Model file for the job. Use its own axes, mm. Face numbers are marked on the shaded views. A direction names the side the tool comes from. Round coordinates to 2 decimals unless told otherwise and drop trailing zeros. Order: outer loops, then holes, each group sorted by start corner. A loop starts at its lowest first (then second) coordinate and runs counter-clockwise, first axis right, second up. Notation, with made-up numbers: M -16,-15.75 L 11,-15.75 A22 cw 11,6.25 Z; hole C 85,12.25 d7. An arc over 180 degrees is marked long. Return JSON: item names as keys, results as strings. Group by question number.
Item 1: Slice it at C-C on x = 15.25. Write the cut outline in (y, z) (3 decimals), then the cut area to 3 significant figures.
Item 2: Pull direction Z, two halves, no side cores. Call the marked faces 1, 2 and 3: pulls with the +Z half, pulls with the -Z half, needs draft (parallel to the pull), parting line crosses it, or undercut.
Item 3: Pin check, flat tips, straight feed: pin 1 Ø1 at (x, y) = (7, -11.5) entering from +Z; pin 2 Ø0.7 at (x, y) = (8.5, 12) entering from +Z; pin 3 Ø2 at (x, z) = (14.5, 8.5) entering from -Y. Stop position of each tip, or through.
Item 4: Slice it at B-B on z = 0. Write the cut outline in (x, y).
Item 5: Slice it at A-A on y = 0. Write the cut outline in (x, z), then the cut area to 3 significant figures.
Item 6: Which spindle directions (+Z, -Z, +X, -X, +Y, -Y) get a long thin tool onto all of the face, cutting with end or side? Do the marked faces 4 and 5. Say none if no direction does.
Item 7: Probe line 1 along Z through (x, y) = (15.25, -8); line 2 along Z through (x, y) = (6.5, 11.5) (3 decimals); line 3 along Z through (x, y) = (12.25, -10). List the from-to ranges inside material, lowest first.
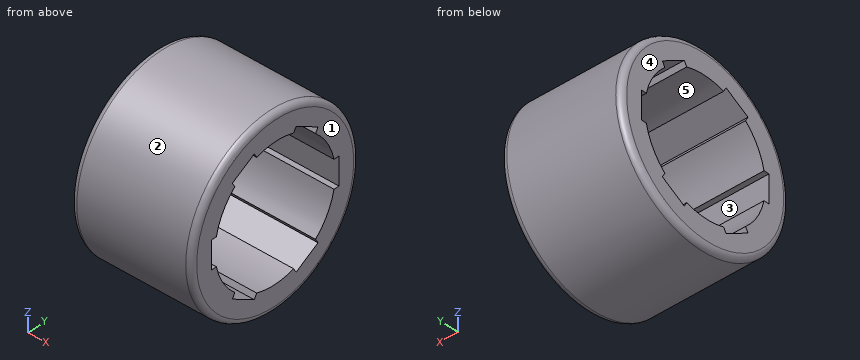
from build123d import *

# Parameters (mm, degrees)
CROQUIS1_R              = 16
SALIENTE_EXTRUIR1_DEPTH = 21
REDONDEO1_R             = 1


with BuildPart() as part:
    # Croquis1 → Saliente-Extruir1 (new body)
    with BuildSketch(Plane(origin=(0, 0, 0), x_dir=(0, 0, -1), z_dir=(1, 0, 0))):
        with Locations(Location((0, 0, 0), (0, 0, 180))):
            Circle(CROQUIS1_R)
        with BuildLine():
            Line((9.340689418, 8.18145135), (11.755689418, 3.99854865))
            Line((11.755689418, 3.99854865), (10.944713731, 3.530331619))
            ThreePointArc((10.944713731, 3.530331619), (11.5, 0), (10.944713731, -3.530331619))
            Line((10.944713731, -3.530331619), (11.755689418, -3.99854865))
            Line((11.755689418, -3.99854865), (9.340689418, -8.18145135))
            Line((9.340689418, -8.18145135), (8.529713731, -7.713234319))
            ThreePointArc((8.529713731, -7.713234319), (5.75, -9.959292144), (2.415, -11.243565938))
            Line((2.415, -11.243565938), (2.415, -12.18))
            Line((2.415, -12.18), (-2.415, -12.18))
            Line((-2.415, -12.18), (-2.415, -11.243565938))
            ThreePointArc((-2.415, -11.243565938), (-5.75, -9.959292144), (-8.529713731, -7.713234319))
            Line((-8.529713731, -7.713234319), (-9.340689418, -8.18145135))
            Line((-9.340689418, -8.18145135), (-11.755689418, -3.99854865))
            Line((-11.755689418, -3.99854865), (-10.944713731, -3.530331619))
            ThreePointArc((-10.944713731, -3.530331619), (-11.5, 0), (-10.944713731, 3.530331619))
            Line((-10.944713731, 3.530331619), (-11.755689418, 3.99854865))
            Line((-11.755689418, 3.99854865), (-9.340689418, 8.18145135))
            Line((-9.340689418, 8.18145135), (-8.529713731, 7.713234319))
            ThreePointArc((-8.529713731, 7.713234319), (-5.75, 9.959292144), (-2.415, 11.243565938))
            Line((-2.415, 11.243565938), (-2.415, 12.18))
            Line((-2.415, 12.18), (2.415, 12.18))
            Line((2.415, 12.18), (2.415, 11.243565938))
            ThreePointArc((2.415, 11.243565938), (5.75, 9.959292144), (8.529713731, 7.713234319))
            Line((8.529713731, 7.713234319), (9.340689418, 8.18145135))
        make_face(mode=Mode.SUBTRACT)
    extrude(amount=SALIENTE_EXTRUIR1_DEPTH)

    # Redondeo1
    redondeo1_edges = [part.edges().sort_by_distance(p)[0] for p in [
        (0, 0, -16),
        (21, 0, -16),
    ]]
    fillet(redondeo1_edges, radius=REDONDEO1_R)


solid = part.part
Output values:
{
 "1": {"outline": "C 0,0 d32; hole M -12.18,-2.415 L -11.244,-2.415 A11.5 ccw -7.713,-8.53 L -8.181,-9.341 L -3.999,-11.756 L -3.53,-10.945 A11.5 ccw 3.53,-10.945 L 3.999,-11.756 L 8.181,-9.341 L 7.713,-8.53 A11.5 ccw 11.244,-2.415 L 12.18,-2.415 L 12.18,2.415 L 11.244,2.415 A11.5 ccw 7.713,8.53 L 8.181,9.341 L 3.999,11.756 L 3.53,10.945 A11.5 ccw -3.53,10.945 L -3.999,11.756 L -8.181,9.341 L -7.713,8.53 A11.5 ccw -11.244,2.415 L -12.18,2.415 Z", "area": "367 mm²"},
 "2": {"face 1": "needs draft", "face 2": "parting line crosses it", "face 3": "undercut"},
 "3": {"pin 1": "z = 11.62", "pin 2": "z = 10.97", "pin 3": "y = -14.13"},
 "4": {"outline": "M 0,-15 A1 ccw 1,-16 L 20,-16 A1 ccw 21,-15 L 21,-12.18 L 0,-12.18 Z; M 0,12.18 L 21,12.18 L 21,15 A1 ccw 20,16 L 1,16 A1 ccw 0,15 Z"},
 "5": {"outline": "M 0,-15 A1 ccw 1,-16 L 20,-16 A1 ccw 21,-15 L 21,-11.5 L 0,-11.5 Z; M 0,11.5 L 21,11.5 L 21,15 A1 ccw 20,16 L 1,16 A1 ccw 0,15 Z", "area": "188 mm²"},
 "6": {"face 4": "+Z, -Z, -X, +Y, -Y", "face 5": "+X, -X"},
 "7": {"line 1": "-13.86 to -9.45, -9.03 to -8.26, 8.26 to 9.03, 9.45 to 13.86", "line 2": "-11.124 to -2.415, 2.415 to 11.124", "line 3": "-12.49 to -5.68, 5.68 to 12.49"}
}
